from build123d import *

# Parameters (mm, degrees)
F0_R     = 9
F0_R_2   = 4.5
F0_W     = 3
F0_H     = 30
F1_DEPTH = 4
F2_R     = 1
F3_R     = 1
F4_R     = 1
F5_R     = 1


with BuildPart() as f1:
    # F0 (on Top) → F1 (new body)
    with BuildSketch(Plane.XY):
        with BuildLine():
            Line((71, -88), (106, -88))
            ThreePointArc((106, -88), (113.071068, -85.071068), (116, -78))
            Line((116, -78), (116, -24))
            Line((116, -24), (127.5, -24))
            ThreePointArc((127.5, -24), (134.571068, -21.071068), (137.5, -14))
            Line((137.5, -14), (137.5, 14))
            ThreePointArc((137.5, 14), (134.571068, 21.071068), (127.5, 24))
            Line((127.5, 24), (116, 24))
            Line((116, 24), (116, 78))
            ThreePointArc((116, 78), (113.071068, 85.071068), (106, 88))
            Line((106, 88), (71, 88))
            Line((71, 88), (71, 103))
            ThreePointArc((71, 103), (70.12132, 105.12132), (68, 106))
            Line((68, 106), (56, 106))
            ThreePointArc((56, 106), (53.87868, 105.12132), (53, 103))
            Line((53, 103), (53, 88))
            Line((53, 88), (-53, 88))
            Line((-53, 88), (-53, 103))
            ThreePointArc((-53, 103), (-53.87868, 105.12132), (-56, 106))
            Line((-56, 106), (-68, 106))
            ThreePointArc((-68, 106), (-70.12132, 105.12132), (-71, 103))
            Line((-71, 103), (-71, 88))
            Line((-71, 88), (-106, 88))
            ThreePointArc((-106, 88), (-113.071068, 85.071068), (-116, 78))
            Line((-116, 78), (-116, 24))
            Line((-116, 24), (-127.5, 24))
            ThreePointArc((-127.5, 24), (-134.571068, 21.071068), (-137.5, 14))
            Line((-137.5, 14), (-137.5, -14))
            ThreePointArc((-137.5, -14), (-134.571068, -21.071068), (-127.5, -24))
            Line((-127.5, -24), (-116, -24))
            Line((-116, -24), (-116, -78))
            ThreePointArc((-116, -78), (-113.071068, -85.071068), (-106, -88))
            Line((-106, -88), (-71, -88))
            Line((-71, -88), (-71, -103))
            ThreePointArc((-71, -103), (-70.12132, -105.12132), (-68, -106))
            Line((-68, -106), (-56, -106))
            ThreePointArc((-56, -106), (-53.87868, -105.12132), (-53, -103))
            Line((-53, -103), (-53, -88))
            Line((-53, -88), (53, -88))
            Line((53, -88), (53, -103))
            ThreePointArc((53, -103), (53.87868, -105.12132), (56, -106))
            Line((56, -106), (68, -106))
            ThreePointArc((68, -106), (70.12132, -105.12132), (71, -103))
            Line((71, -103), (71, -88))
        make_face()
        with Locations((-78, -58)):
            Circle(F0_R, mode=Mode.SUBTRACT)
        with Locations((-62, -97)):
            Circle(F0_R_2, mode=Mode.SUBTRACT)
        with Locations((-39, -58)):
            Circle(F0_R, mode=Mode.SUBTRACT)
        with Locations((-78, -23)):
            Circle(F0_R, mode=Mode.SUBTRACT)
        with Locations((-39, -23)):
            Circle(F0_R, mode=Mode.SUBTRACT)
        with Locations((62, -97)):
            Circle(F0_R_2, mode=Mode.SUBTRACT)
        with Locations((0, -58)):
            Circle(F0_R, mode=Mode.SUBTRACT)
        with Locations((39, -58)):
            Circle(F0_R, mode=Mode.SUBTRACT)
        with Locations((78, -58)):
            Circle(F0_R, mode=Mode.SUBTRACT)
        with Locations((0, -23)):
            Circle(F0_R, mode=Mode.SUBTRACT)
        with Locations((39, -23)):
            Circle(F0_R, mode=Mode.SUBTRACT)
        with Locations((78, -23)):
            Circle(F0_R, mode=Mode.SUBTRACT)
        Polygon((-127.5, 15), (-127.5, 0), (-127.5, -15), (-130.5, -15), (-130.5, 0), (-130.5, 15), align=None, mode=Mode.SUBTRACT)
        with Locations((-78, 12)):
            Circle(F0_R, mode=Mode.SUBTRACT)
        with Locations((-78, 47)):
            Circle(F0_R, mode=Mode.SUBTRACT)
        with Locations((-39, 12)):
            Circle(F0_R, mode=Mode.SUBTRACT)
        with Locations((-39, 47)):
            Circle(F0_R, mode=Mode.SUBTRACT)
        with Locations((-62, 97)):
            Circle(F0_R_2, mode=Mode.SUBTRACT)
        with Locations((0, 12)):
            Circle(F0_R, mode=Mode.SUBTRACT)
        with Locations((39, 12)):
            Circle(F0_R, mode=Mode.SUBTRACT)
        with Locations((0, 47)):
            Circle(F0_R, mode=Mode.SUBTRACT)
        with Locations((39, 47)):
            Circle(F0_R, mode=Mode.SUBTRACT)
        with Locations((78, 12)):
            Circle(F0_R, mode=Mode.SUBTRACT)
        with Locations((110, 0)):
            Circle(F0_R, mode=Mode.SUBTRACT)
        with Locations((129, 0)):
            Rectangle(F0_W, F0_H, mode=Mode.SUBTRACT)
        with Locations((78, 47)):
            Circle(F0_R, mode=Mode.SUBTRACT)
        with Locations((62, 97)):
            Circle(F0_R_2, mode=Mode.SUBTRACT)
    extrude(amount=F1_DEPTH)

    # F2
    f2_edges = [f1.edges().sort_by_distance(p)[0] for p in [
        (127.5, -15, 2),
        (130.5, -15, 2),
    ]]
    fillet(f2_edges, radius=F2_R)

    # F3
    f3_edges = [f1.edges().sort_by_distance(p)[0] for p in [
        (127.5, 15, 2),
        (130.5, 15, 2),
    ]]
    fillet(f3_edges, radius=F3_R)

    # F4
    f4_edges = [f1.edges().sort_by_distance(p)[0] for p in [
        (-130.5, 15, 2),
        (-127.5, 15, 2),
    ]]
    fillet(f4_edges, radius=F4_R)

    # F5
    f5_edges = [f1.edges().sort_by_distance(p)[0] for p in [
        (-130.5, -15, 2),
        (-127.5, -15, 2),
    ]]
    fillet(f5_edges, radius=F5_R)


solid = f1.part
Read the model definition and answer for the solid it produces. Units are mm, in the model's axes. Coordinates: 2 decimals unless noted, no trailing zeros. Order: outer loops, then holes, each group sorted by start corner. A loop starts at its lowest first (then second) coordinate and runs counter-clockwise, first axis right, second up. Notation, with made-up numbers: M 51,72.5 L 74,72.5 A13 ccw 74,79.5 Z; hole C 38.5,33.5 d11. An arc over 180 degrees is marked long. Put each result on its own line as item: value. Start each with the question number.
Item 1: Section B-B, the plane x = -61 is taken. Determine the outline of the cut face in (y, z).
Item 2: Section A-A, the plane y = -97 is taken. Determine the outline of the cut face in (x, z).
Item 3: Given pin 1 Ø1.2 at (y, z) = (92.5, 2.5) entering from +X; pin 2 Ø2 at (y, z) = (30.5, 1) entering from -X; pin 3 Ø2 at (y, z) = (95.5, 2) entering from -X; pin 4 Ø14.5 at (x, y) = (39, -58) entering from +Z, each flat-ended and moving along its own axis, determine where each tip first touches the part or whether it passes through.
Item 4: Section C-C, the plane x = 80 is taken. Determine the outline of the cut face in (y, z).
Item 5: Section D-D, the plane z = 0.7 is taken. Count the separate pieces of the cut face and the enclosed holes in it, plus the area to 3 significant figures.
Item 6: Consider probe 1 along Y at (x, z) = (0, 2.75); probe 2 along X at (y, z) = (90, 3.45); probe 3 along X at (y, z) = (-53, 0.8). Determine where each line is inside the solid, lowest interval first. Write a range as [from, to].
Item 7: The mould has two halves that part along X. Classify faces 1 (the face through (118.584, 2.703, 1.972)), 2 (the face through (-113.15, -84.99, 1.97)), 3 (the face through (134.65, 20.99, 1.97)): +X half, -X half, draft (parallel to the pull), parting line (faces both ways), or undercut.
Computed:
1. outline: M -106,0 L -101.39,0 L -101.39,4 L -106,4 Z; M -92.61,0 L 92.61,0 L 92.61,4 L -92.61,4 Z; M 101.39,0 L 106,0 L 106,4 L 101.39,4 Z
2. outline: M -71,0 L -66.5,0 L -66.5,4 L -71,4 Z; M -57.5,0 L -53,0 L -53,4 L -57.5,4 Z; M 53,0 L 57.5,0 L 57.5,4 L 53,4 Z; M 66.5,0 L 71,0 L 71,4 L 66.5,4 Z
3. pin 1: stops at x = 71
3. pin 2: stops at x = -116
3. pin 3: stops at x = -71
3. pin 4: passes through
4. outline: M -88,0 L -66.77,0 L -66.77,4 L -88,4 Z; M -49.23,0 L -31.77,0 L -31.77,4 L -49.23,4 Z; M -14.23,0 L 3.23,0 L 3.23,4 L -14.23,4 Z; M 20.77,0 L 38.23,0 L 38.23,4 L 20.77,4 Z; M 55.77,0 L 88,0 L 88,4 L 55.77,4 Z
5. separate pieces: 1
5. enclosed holes: 27
5. area: 38,200 mm2
6. probe 1: y = [-88, -67], [-49, -32], [-14, 3], [21, 38], [56, 88]
6. probe 2: x = [-71, -53], [53, 71]
6. probe 3: x = [-116, -85.48], [-70.52, -46.48], [-31.52, -7.48], [7.48, 31.52], [46.48, 70.52], [85.48, 116]
7. face 1: undercut
7. face 2: -X half
7. face 3: +X half
